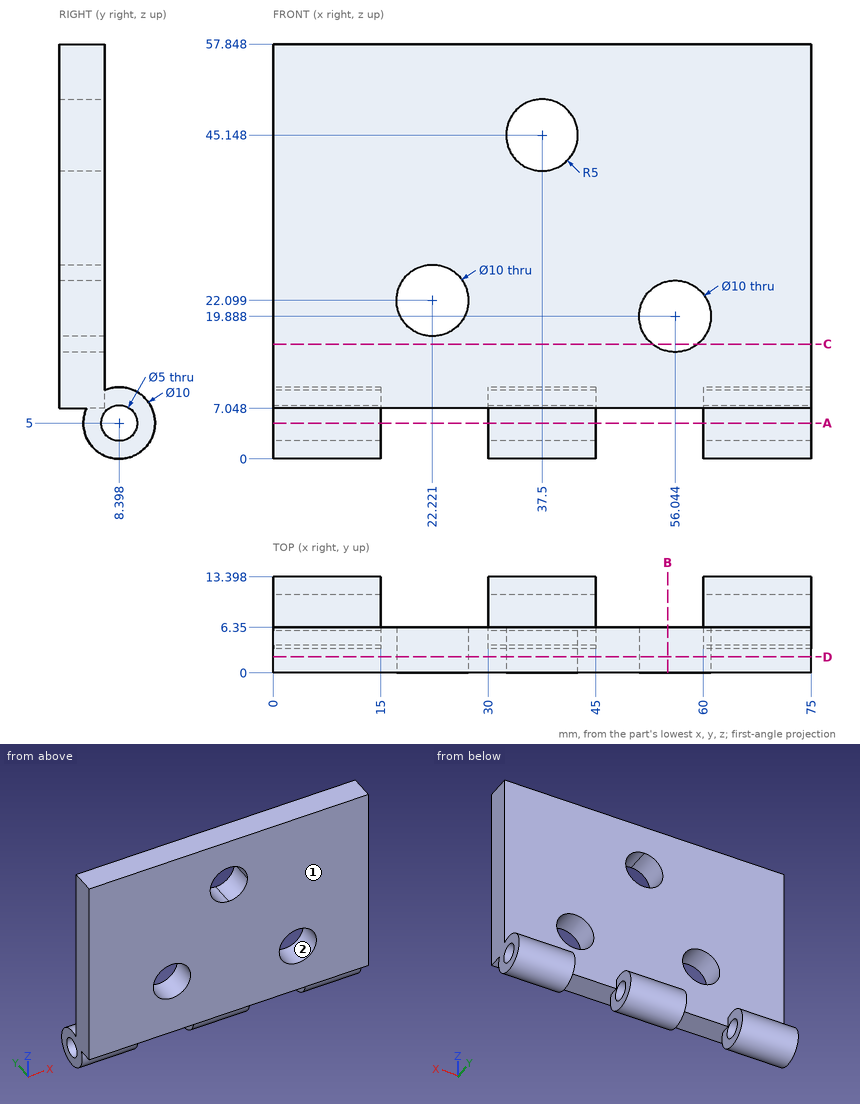
Could you check a few things on this drawing? It's one solid part, dimensions in mm from its lowest x, y, z. Coordinates: 2 decimals unless noted, no trailing zeros. Write each loop counter-clockwise with the first axis right and the second up, starting at its lowest first coordinate (ties: lowest second). Pieces come first, ordered by that corner, then holes.
1) If we section it at A-A (z = 5): List the corners of the cut face in (x, y) for me, plus the area to 3 significant figures.
Filled in:
outline: (0, 3.4) - (15, 3.4) - (15, 5.9) - (0, 5.9) - close; (0, 10.9) - (15, 10.9) - (15, 13.4) - (0, 13.4) - close; (30, 3.4) - (45, 3.4) - (45, 5.9) - (30, 5.9) - close; (30, 10.9) - (45, 10.9) - (45, 13.4) - (30, 13.4) - close; (60, 3.4) - (75, 3.4) - (75, 5.9) - (60, 5.9) - close; (60, 10.9) - (75, 10.9) - (75, 13.4) - (60, 13.4) - close
area: 225 mm2
2) If we section it at C-C (z = 16): List the corners of the cut face in (x, y) for me.
Filled in:
outline: (0, 0) - (52.9, 0) - (52.9, 6.35) - (0, 6.35) - close; (59.19, 0) - (75, 0) - (75, 6.35) - (59.19, 6.35) - close
3) Thinking about a two-plate mould opening in X: for the marked faces 1 and 2, which applies, +X half, -X half, draft (parallel to the pull), parting line (faces both ways), or undercut?
Filled in:
face 1: draft
face 2: undercut
4) I'm going to push flat-ended pins straight in: pin 1 (3 mm diameter, centred on x = 25.5, y = 8.5, fed in from +Z); pin 2 (1 mm diameter, centred on x = 57.5, z = 52, fed in from +Y); pin 3 (5 mm diameter, centred on x = 40.5, y = 3.5, fed in from -Z). Where does each tip first touch, or does it pass through?
Filled in:
pin 1: passes through
pin 2: stops at y = 6.35
pin 3: stops at z = 0.61
5) If we section it at D-D (y = 2.25): List the corners of the cut face in (x, z) for me, plus the area to 3 significant figures.
Filled in:
outline: (0, 7.05) - (75, 7.05) - (75, 57.85) - (0, 57.85) - close; hole circle Ø10 at (22.22, 22.1); hole circle Ø10 at (37.5, 45.15); hole circle Ø10 at (56.04, 19.89)
area: 3,570 mm2
6) If we section it at B-B (x = 55): List the corners of the cut face in (y, z) for me.
Filled in:
outline: (0, 7.05) - (6.35, 7.05) - (6.35, 15) - (0, 15) - close; (0, 24.78) - (6.35, 24.78) - (6.35, 57.85) - (0, 57.85) - close
7) If I drill on line 1 (Y direction, x = 64, z = 5); line 2 (X direction, y = 4.75, z = 20) (1 decimal); line 3 (Y direction, x = 54.5, z = 51), over which ranges is the centre line in solid material (lowest first)?
Filled in:
line 1: y = 3.4 to 5.9, 10.9 to 13.4
line 2: x = 0 to 17.7, 26.8 to 51, 61 to 75
line 3: y = 0 to 6.35
